Design review of the part built by this model. Coordinates are the model's own, in mm. A direction names the side the tool comes from. Give positions to 0.01 mm unless a question says otherwise; leave off trailing zeros. Write each loop counter-clockwise with the first axis right and the second up, starting at its lowest first coordinate (ties: lowest second). Pieces come first, ordered by that corner, then holes. Notation, with made-up numbers: (-37, -34) - (-23, -34) arc R24 cw to (-23, 4) - close; hole circle Ø6 at (50, -17). An arc over 180 degrees is marked (long way). Use a Markdown table: item, result. Add a question column.
```python
from build123d import *

# Parameters (mm, degrees)
SKETCH1_R           = 19.25
BOSS_EXTRUDE1_DEPTH = 41.3
SKETCH3_R           = 1.585
BOSS_EXTRUDE2_DEPTH = 13.3
SKETCH4_R           = 6.5
BOSS_EXTRUDE3_DEPTH = 4.5
SKETCH5_R           = 17.9
BOSS_EXTRUDE4_DEPTH = 13.16
SKETCH6_R           = 5.1
BOSS_EXTRUDE5_DEPTH = 3
SKETCH7_R           = 2.375
BOSS_EXTRUDE6_DEPTH = 3
SKETCH8_R           = 1.6
CUT_EXTRUDE1_DEPTH  = 2.999994


with BuildPart() as part:
    # Sketch1 → Boss-Extrude1 (new body)
    with BuildSketch(Plane.XY):
        Circle(SKETCH1_R)
    extrude(amount=BOSS_EXTRUDE1_DEPTH)

    # Sketch3 → Boss-Extrude2 (add)
    with BuildSketch(Plane.XY.offset(41.3)):
        Circle(SKETCH3_R)
    extrude(amount=BOSS_EXTRUDE2_DEPTH)

    # Sketch4 → Boss-Extrude3 (add)
    with BuildSketch(Plane.XY.offset(41.3)):
        Circle(SKETCH4_R)
    extrude(amount=BOSS_EXTRUDE3_DEPTH)

    # Sketch5 → Boss-Extrude4 (add)
    with BuildSketch(Plane(origin=(0, 0, 0), x_dir=(-1, 0, 0), z_dir=(0, 0, -1))):
        Circle(SKETCH5_R)
    extrude(amount=BOSS_EXTRUDE4_DEPTH)

    # Sketch6 → Boss-Extrude5 (add)
    with BuildSketch(Plane(origin=(0, 0, -13.16), x_dir=(-1, 0, 0), z_dir=(0, 0, -1))):
        Circle(SKETCH6_R)
    extrude(amount=BOSS_EXTRUDE5_DEPTH)

    # Sketch7 → Boss-Extrude6 (add)
    with BuildSketch(Plane(origin=(0, 0, -16.16), x_dir=(-1, 0, 0), z_dir=(0, 0, -1))):
        Circle(SKETCH7_R)
    extrude(amount=BOSS_EXTRUDE6_DEPTH)

    # Sketch8 → Cut-Extrude1 (cut)
    with BuildSketch(Plane.XY.offset(41.3)):
        with Locations((0, 12.5)):
            Circle(SKETCH8_R)
        with Locations((0, -12.5)):
            Circle(SKETCH8_R)
    extrude(amount=-CUT_EXTRUDE1_DEPTH, mode=Mode.SUBTRACT)


solid = part.part
```
(1) Insertion check: pin 1 (1.6 mm diameter, centred on x = -0.5, y = 12, fed in from +Z); pin 2 (1 mm diameter, centred on y = -10.5, z = -5, fed in from +X); pin 3 (6 mm diameter, centred on x = -9, y = -1.5, fed in from +Z). Each pin has a flat end and moves straight along its axis. Give the tip position at first contact, or say it passes through.
(2) Tool access review of faces 1 (the face through (-1.26, -0.96, 50.14)), 2 (the face through (0, 0, 54.6)), 3 (the face through (-1.1, 2.3, -16.16)): name each direction out of +Z, -Z, +X, -X, +Y, -Y from which nothing blocks a thin tool from reaching the whole face with its end or side.
(3) Add section D-D (y = 16). State the section outline as (x, z) points, and give its area (3 significant figures).
(4) Add section B-B (y = 0). State the section outline as (x, z) points (3 decimals), and give its area (3 significant figures).
(5) For line 1 along Y through (x, z) = (0, 39); line 2 along Z through (x, y) = (6.5, -7); line 3 along Z through (x, y) = (-1, 2), list the stretches that pass through material, from the lowest coordinate up.
(6) Mouldability with a two-part tool opening along Y and no side actions: class faces 4 (the face through (-15.28, -11.71, 20.36)), 5 (the face through (0, -12, 38.3)), 6 (the face through (0, -8, 41.3)) as +Y half, -Y half, draft (parallel to the pull), parting line (faces both ways), or undercut.
(7) Add section C-C (z = 8.5). State the section outline as (x, y) points.
Answers follow:
| question | item | result |
|---|---|---|
| 1 | pin 1 | z = 38.3 |
| 1 | pin 2 | x = 14.85 |
| 1 | pin 3 | z = 45.8 |
| 2 | face 1 | +Z |
| 2 | face 2 | +Z, +X, -X, +Y, -Y |
| 2 | face 3 | -Z |
| 3 | outline | (-10.7, 0) - (-8.03, 0) - (-8.03, -13.16) - (8.03, -13.16) - (8.03, 0) - (10.7, 0) - (10.7, 41.3) - (-10.7, 41.3) - close |
| 3 | area | 1,100 mm^2 |
| 4 | outline | (-19.25, 0) - (-17.9, 0) - (-17.9, -13.16) - (-5.1, -13.16) - (-5.1, -16.16) - (-2.375, -16.16) - (-2.375, -19.16) - (2.375, -19.16) - (2.375, -16.16) - (5.1, -16.16) - (5.1, -13.16) - (17.9, -13.16) - (17.9, 0) - (19.25, 0) - (19.25, 41.3) - (6.5, 41.3) - (6.5, 45.8) - (1.585, 45.8) - (1.585, 54.6) - (-1.585, 54.6) - (-1.585, 45.8) - (-6.5, 45.8) - (-6.5, 41.3) - (-19.25, 41.3) - close |
| 4 | area | 2,190 mm^2 |
| 5 | line 1 | -19.25 to -14.1, -10.9 to 10.9, 14.1 to 19.25 |
| 5 | line 2 | -13.16 to 41.3 |
| 5 | line 3 | -19.16 to 45.8 |
| 6 | face 4 | parting line |
| 6 | face 5 | undercut |
| 6 | face 6 | draft |
| 7 | outline | circle Ø38.5 at (0, 0) |
